from build123d import *

# Parameters (mm, degrees)
SKETCH1_R               = 4
BOSS_EXTRUDE1_DEPTH     = 2
SKETCH2_W               = 25
SKETCH2_H               = 430
BOSS_EXTRUDE2_DEPTH     = 2
SKETCH3_R               = 3.3
CUT_EXTRUDE1_DEPTH      = 1
CUT_EXTRUDE1_DEPTH_BACK = 36.499546541


with BuildPart() as part:
    # Sketch1 → Boss-Extrude1 (new body)
    with BuildSketch(Plane.YZ):
        Polygon((15, 230), (15, -200), (0, -200), (0, -24.43744304), (-10, -14.43744304), (-10, 25), (-18.499546541, 25), (-18.499546541, 55), (-10, 55), (-10, 230), align=None)
        Circle(SKETCH1_R, mode=Mode.SUBTRACT)
        with Locations((-3.499546541, 40)):
            Circle(SKETCH1_R, mode=Mode.SUBTRACT)
    extrude(amount=-BOSS_EXTRUDE1_DEPTH)

    # Sketch2 → Boss-Extrude2 (add)
    with BuildSketch(Plane(origin=(0, 15, 0), x_dir=(-1, 0, 0), z_dir=(0, 1, 0))):
        with Locations((12.5, 15)):
            Rectangle(SKETCH2_W, SKETCH2_H)
    extrude(amount=BOSS_EXTRUDE2_DEPTH)

    # Mirror1: part across plane


with BuildPart() as part_1:
    add(part.part)
    add(part.part.mirror(Plane(origin=(-25, 17, 230), x_dir=(0, 0, 1), z_dir=(1, 0, 0))))

    # Sketch3 → Cut-Extrude1 (cut, two sides)
    with BuildSketch(Plane(origin=(0, 17, 0), x_dir=(-1, 0, 0), z_dir=(0, 1, 0))) as cut_extrude1_sk:
        with Locations((25, 200)):
            Circle(SKETCH3_R)
        with Locations((25, -170)):
            Circle(SKETCH3_R)
    extrude(amount=CUT_EXTRUDE1_DEPTH, mode=Mode.SUBTRACT)
    extrude(cut_extrude1_sk.sketch, amount=-CUT_EXTRUDE1_DEPTH_BACK, mode=Mode.SUBTRACT)


solid = part_1.part
Here's how the part is built. I have some questions about the finished solid (model axes, mm). A direction names the side the tool comes from. Give positions to 0.01 mm unless a question says otherwise; leave off trailing zeros. Order: outer loops, then holes, each group sorted by start corner. A loop starts at its lowest first (then second) coordinate and runs counter-clockwise, first axis right, second up. Notation, with made-up numbers: (43.25, 19) -> (85.25, 19) arc R19 cw to (85.25, 50) -> close; hole circle Ø3 at (15, 24.5). An arc over 180 degrees is marked (long way). Use a Markdown table: item, result. Add a question column.
Item 1: I need wall thicknesses on line 1 (Z direction, x = -25, y = 15.5); line 2 (X direction, y = -0.5, z = 26); line 3 (Y direction, x = -7, z = 81.5). Which ranges of each line are inside material? Lowest first, please.
Item 2: Will these pins go through, and if not, where does the flat tip stop? pin 1 (1.6 mm diameter, centred on x = -1, y = -15.5, fed in from -Z); pin 2 (0.6 mm diameter, centred on x = -1, y = -14, fed in from +Z); pin 3 (2 mm diameter, centred on x = -49, z = -115, fed in from -Y).
Item 3: Imagine slicing it at B-B on x = -14.5. Please give me the cut outline in (y, z).
Item 4: For faces 1 (the face through (-25, 15, 18)), 2 (the face through (-24.28, 16.01, 196.78)), which set-ups out of +Z, -Z, +X, -X, +Y, -Y let a thin tool reach every point of the face, with its end or its side?
Item 5: Imagine slicing it at A-A on z = 40. Please give me the cut outline in (x, y).
Item 6: If we mould it in two halves opening along X, with no side actions, what happens to faces 3 (the face through (-50, 3, 60)), 4 (the face through (-48, 2, 66)), 5 (the face through (-0.986, -0.867, -3.905))? For each: pulls with the +X half, pulls with the -X half, needs draft (parallel to the pull), parting line crosses it, or undercut.
Data:
| question | item | result |
|---|---|---|
| 1 | line 1 | z = -200 to -173.3, -166.7 to 196.7, 203.3 to 230 |
| 1 | line 2 | x = -50 to -48, -2 to 0 |
| 1 | line 3 | y = 15 to 17 |
| 2 | pin 1 | stops at z = 25 |
| 2 | pin 2 | stops at z = 55 |
| 2 | pin 3 | stops at y = 0 |
| 3 | outline | (15, -200) -> (17, -200) -> (17, 230) -> (15, 230) -> close |
| 4 | face 1 | +Z, -Z, -Y |
| 4 | face 2 | +Y, -Y |
| 5 | outline | (-50, -18.5) -> (-48, -18.5) -> (-48, -7.5) -> (-50, -7.5) -> close; (-50, 0.5) -> (-48, 0.5) -> (-48, 15) -> (-2, 15) -> (-2, 0.5) -> (0, 0.5) -> (0, 17) -> (-50, 17) -> close; (-2, -18.5) -> (0, -18.5) -> (0, -7.5) -> (-2, -7.5) -> close |
| 6 | face 3 | pulls with the -X half |
| 6 | face 4 | undercut |
| 6 | face 5 | needs draft |
